```python
from build123d import *

# Parameters (mm, degrees)
F1_DEPTH = 1
F2_R     = 3.6
F2_R_2   = 2.9
F3_DEPTH = 5
F4_DEPTH = 1


with BuildPart() as f1:
    # F0 (on Front) → F1 (new body, symmetric)
    with BuildSketch(Plane.XZ):
        with BuildLine():
            ThreePointArc((3.8359832735, -2.3527074457), (4.3308154389, -1.2223083222), (4.5, 0))
            ThreePointArc((4.5, 0), (4.3308154389, 1.2223083222), (3.8359832735, 2.3527074457))
            ThreePointArc((3.8359832735, 2.3527074457), (-4.5, 0), (3.8359832735, -2.3527074457))
        make_face()
        with BuildLine():
            ThreePointArc((3.8359832735, 2.3527074457), (4.3308154389, 1.2223083222), (4.5, 0))
            ThreePointArc((4.5, 0), (4.3308154389, -1.2223083222), (3.8359832735, -2.3527074457))
            Line((3.8359832735, -2.3527074457), (59.7996972501, -0.2551520593))
            Line((59.7996972501, -0.2551520593), (59.9825401634, -9.9e-09))
            Line((59.9825401634, -9.9e-09), (59.7996972501, 0.2551520395))
            Line((59.7996972501, 0.2551520395), (3.8359832735, 2.3527074457))
        make_face()
    extrude(amount=F1_DEPTH, both=True)

    # F2 (on face) → F3 (join)
    with BuildSketch(Plane(origin=(0, 1, 0), x_dir=(-1, 0, 0), z_dir=(0, 1, 0))):
        Circle(F2_R)
        Circle(F2_R_2, mode=Mode.SUBTRACT)
    extrude(amount=-F3_DEPTH)

    # F0 (on Front) → F4 (join, symmetric)
    with BuildSketch(Plane.XZ):
        with BuildLine():
            ThreePointArc((3.8359832735, 2.3527074457), (4.3308154389, 1.2223083222), (4.5, 0))
            ThreePointArc((4.5, 0), (4.3308154389, -1.2223083222), (3.8359832735, -2.3527074457))
            Line((3.8359832735, -2.3527074457), (59.7996972501, -0.2551520593))
            Line((59.7996972501, -0.2551520593), (59.9825401634, -9.9e-09))
            Line((59.9825401634, -9.9e-09), (59.7996972501, 0.2551520395))
            Line((59.7996972501, 0.2551520395), (3.8359832735, 2.3527074457))
        make_face()
    extrude(amount=F4_DEPTH, both=True)


solid = f1.part
```
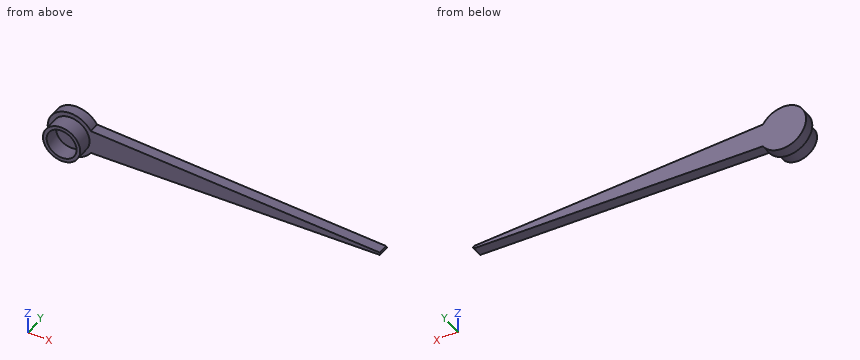
Check sheet for the modelled part. Datum: model origin and axes. Units: mm. Round coordinates to 2 decimals unless told otherwise and drop trailing zeros. Order: outer loops, then holes, each group sorted by start corner. A loop starts at its lowest first (then second) coordinate and runs counter-clockwise, first axis right, second up.
1) Scan lines: line 1 (Z direction, x = 0, y = -1.8); line 2 (X direction, y = -3.4, z = 0.25); line 3 (X direction, y = -3.15, z = -2.5). Record each from-to range of solid material in increasing order.
2) Section check C-C (x = 53). Record the boundary of the cut face in (y, z), and give its area (3 significant figures).
3) Go/stop test with flat-tipped pins: pin 1 Ø1 at (x, z) = (34.5, 2.5) entering from -Y; pin 2 Ø4.5 at (x, z) = (26.5, -0.5) entering from -Y; pin 3 Ø1 at (y, z) = (0.5, -3) entering from +X. Record where each tip stops, or that it passes through.
4) Section check D-D (x = 19.5). Record the boundary of the cut face in (y, z).
5) Section check A-A (x = 0). Record the boundary of the cut face in (y, z).
6) Section check B-B (y = -2.3). Record the boundary of the cut face in (x, z).
Result:
1. line 1: z = -3.6 to -2.9, 2.9 to 3.6
1. line 2: x = -3.59 to -2.89, 2.89 to 3.59
1. line 3: x = -2.59 to -1.47, 1.47 to 2.59
2. outline: (-1, -0.51) - (1, -0.51) - (1, 0.51) - (-1, 0.51) - close
2. area: 2.04 mm2
3. pin 1: passes through
3. pin 2: stops at y = -1
3. pin 3: stops at x = 3.74
4. outline: (-1, -1.77) - (1, -1.77) - (1, 1.77) - (-1, 1.77) - close
5. outline: (-4, -3.6) - (-1, -3.6) - (-1, -4.5) - (1, -4.5) - (1, 4.5) - (-1, 4.5) - (-1, 3.6) - (-4, 3.6) - (-4, 2.9) - (-1, 2.9) - (-1, -2.9) - (-4, -2.9) - close
6. outline: circle Ø7.2 at (0, 0); hole circle Ø5.8 at (0, 0)
